```python
from build123d import *

# Parameters (mm, degrees)
BOSS_EXTRUDE1_DEPTH = 325
FILLET1_R           = 1


with BuildPart() as part:
    # Sketch2 → Boss-Extrude1 (new body)
    with BuildSketch(Plane(origin=(0, 0, 0), x_dir=(0, 0, -1), z_dir=(1, 0, 0))):
        with BuildLine():
            Line((2.5, 5.837165408), (2.5, 4.35))
            Line((2.5, 4.35), (-2.5, 4.35))
            Line((-2.5, 4.35), (-2.5, 5.837165408))
            ThreePointArc((-2.5, 5.837165408), (0, -6.35), (2.5, 5.837165408))
        make_face()
    extrude(amount=BOSS_EXTRUDE1_DEPTH)

    # Fillet1
    fillet1_edges = [part.edges().sort_by_distance(p)[0] for p in [
        (0, -6.35, 0),
        (325, -6.35, 0),
    ]]
    fillet(fillet1_edges, radius=FILLET1_R)


solid = part.part
```
Geometry check sheet. Reference: the model listing, model coordinates, mm. Coordinates: 2 decimals unless noted, no trailing zeros. Write each loop counter-clockwise with the first axis right and the second up, starting at its lowest first coordinate (ties: lowest second). Pieces come first, ordered by that corner, then holes. Notation, with made-up numbers: M 88.25,-35 L 136.25,-35 A22 ccw 136.25,-22 Z; hole C 87.5,46.5 d3. An arc over 180 degrees is marked long. One line per item, written item: value. Start each with the question number.
(1) Sectioned sample at B-B, the plane x = 115. Enter the section's corners in (y, z), and give its area (3 significant figures).
(2) Sectioned sample at A-A, the plane z = 0. Enter the section's corners in (x, y).
(3) Depth check by flat-ended pin: pin 1 (6 mm diameter, centred on x = 260, y = -1, fed in from +Z); pin 2 (1.2 mm diameter, centred on x = 92, y = 5, fed in from +Z); pin 3 (5 mm diameter, centred on x = 195.5, z = -3.5, fed in from -Y); pin 4 (2.5 mm diameter, centred on x = 111.5, z = 0.5, fed in from +Y). Enter the tip coordinate at first touch or a pass-through.
(4) Release check for a two-part mould opening along Z. For faces 1 (the face through (325, 0, 0)), 2 (the face through (160.239, -6.345, 0.243)), 3 (the face through (160, 4.35, 0)) record: released by +Z, released by -Z, zero draft, split by the parting line, or undercut.
(5) Scan lines: line 1 along Z through (x, y) = (71, 5); line 2 along Z through (x, y) = (283, -0.75); line 3 along Z through (x, y) = (203, 5.25). Record each from-to range of solid material in increasing order. Write a range as [from, to].
Filled sheet:
1. outline: M 4.35,-2.5 L 4.35,2.5 L 5.84,2.5 A6.35 ccw long 5.84,-2.5 Z
1. area: 118 mm²
2. outline: M 0,-5.35 A1 ccw 1,-6.35 L 324,-6.35 A1 ccw 325,-5.35 L 325,4.35 L 0,4.35 Z
3. pin 1: z = 6.35
3. pin 2: z = 4.58
3. pin 3: y = -6.27
3. pin 4: y = 4.35
4. face 1: zero draft
4. face 2: split by the parting line
4. face 3: undercut
5. line 1: [-3.91, -2.5], [2.5, 3.91]
5. line 2: [-6.31, 6.31]
5. line 3: [-3.57, -2.5], [2.5, 3.57]
